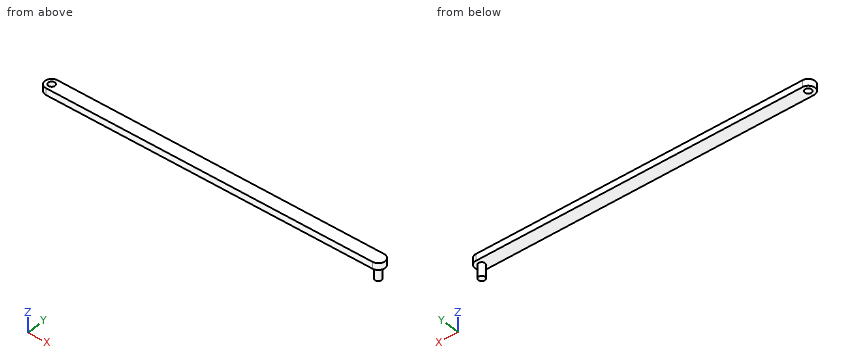
```python
from build123d import *

# Parameters (mm, degrees)
EXTRUDE_1_DEPTH     = 2
SKETCH_2_R          = 1
EXTRUDE_2_DEPTH     = 4
SKETCH_3_R          = 1
CUT_EXTRUDE_1_DEPTH = 4


with BuildPart() as part:
    # 草图1 → 凸台-拉伸1 (new body)
    with BuildSketch(Plane.XY):
        with BuildLine():
            Line((-59.140028095, -2), (40.859971905, -2))
            ThreePointArc((40.859971905, -2), (42.859971905, 0), (40.859971905, 2))
            Line((40.859971905, 2), (-59.140028095, 2))
            ThreePointArc((-59.140028095, 2), (-61.140028095, 0), (-59.140028095, -2))
        make_face()
    extrude(amount=EXTRUDE_1_DEPTH)

    # 草图2 → 凸台-拉伸2 (add)
    with BuildSketch(Plane(origin=(0, 0, 0), x_dir=(-1, 0, 0), z_dir=(0, 0, -1))):
        with Locations((-40.859971905, 0)):
            Circle(SKETCH_2_R)
    extrude(amount=EXTRUDE_2_DEPTH)

    # 草图3 → 切除-拉伸1 (cut)
    with BuildSketch(Plane(origin=(0, 0, 0), x_dir=(-1, 0, 0), z_dir=(0, 0, -1))):
        with Locations((59.140028095, 0)):
            Circle(SKETCH_3_R)
    extrude(amount=-CUT_EXTRUDE_1_DEPTH, mode=Mode.SUBTRACT)


solid = part.part
```
Verification items for the finished model (mm, model axes). Round coordinates to 2 decimals unless told otherwise and drop trailing zeros. Write each loop counter-clockwise with the first axis right and the second up, starting at its lowest first coordinate (ties: lowest second). Pieces come first, ordered by that corner, then holes. Notation, with made-up numbers: (51, 33.25) - (59, 33.25) arc R35 cw to (59, 65.25) - close; hole circle Ø11 at (38.25, 55.5). An arc over 180 degrees is marked (long way). Answer as a JSON object with one key per item and string values. Group by question number.
Q1. Section check A-A, the plane y = 0. Enter the section's corners in (x, z), plus the area to 3 significant figures.
Q2. Section check B-B, the plane x = -38. Enter the section's corners in (y, z), plus the area to 3 significant figures.
Q3. Section check C-C, the plane z = -1.45. Enter the section's corners in (x, y).
Q4. Thickness scan on line 1 (X direction, y = 0.2, z = 1.4); line 2 (Z direction, x = 6.5, y = -0.2); line 3 (X direction, y = -0.1, z = -1.7). Record the ranges inside material, lowest first.
Found:
{
 "1": {"outline": "(-61.14, 0) - (-60.14, 0) - (-60.14, 2) - (-61.14, 2) - close; (-58.14, 0) - (39.86, 0) - (39.86, -4) - (41.86, -4) - (41.86, 0) - (42.86, 0) - (42.86, 2) - (-58.14, 2) - close", "area": "212 mm^2"},
 "2": {"outline": "(-2, 0) - (2, 0) - (2, 2) - (-2, 2) - close", "area": "8.00 mm^2"},
 "3": {"outline": "circle Ø2 at (40.86, 0)"},
 "4": {"line 1": "x = -61.13 to -60.12, -58.16 to 42.85", "line 2": "z = 0 to 2", "line 3": "x = 39.86 to 41.85"}
}
